Can you work these out from the model? Positions are in its coordinate system, mm. Face numbers are marked on the shaded views. A direction names the side the tool comes from. Coordinates: 2 decimals unless noted, no trailing zeros. Write each loop counter-clockwise with the first axis right and the second up, starting at its lowest first coordinate (ties: lowest second). Pieces come first, ordered by that corner, then holes.
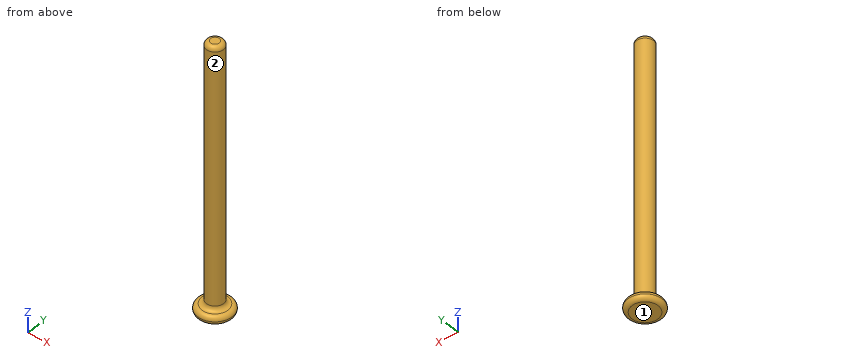
Autodesk Inventor part; units mm, degrees
ref_plane "YZ Plane" through (0, 0, 0) normal (1, 0, 0) x (0, 1, 0)
ref_plane "XZ Plane" through (0, 0, 0) normal (0, 1, 0) x (-1, 0, 0)
ref_plane "XY Plane" through (0, 0, 0) normal (0, 0, 1) x (1, 0, 0)
sketch "Sketch1" plane through (0, 0, 0) normal (0, 0, 1) x (1, 0, 0)
  circle A0 centre (0, 0) radius 2
  dimension "d0" = 4
extrude "Extrusion1" add sketch "Sketch1" along normal blind 1
sketch "Sketch2" plane through (0, 0, 1) normal (0, 0, 1) x (1, 0, 0)
  circle A0 centre (0, 0) radius 1
  dimension "d3" = 2
extrude "Extrusion2" add sketch "Sketch2" along normal blind 30
fillet "Fillet1" radius 0.5 1 edges at (-1, 0, 31)
fillet "Fillet2" radius 0.5 3 edges at (-1, 0, 1) (-2, 0, 1) (-2, 0, 0)
properties part number "ufakpin"
1. If I drill on L1, parallel to Y at x = -0.1, z = 23.5; L2, parallel to Z at x = 1.2, y = -0.75; L3, parallel to Z at x = 1.15, y = -0.2, over which ranges is the centre line in solid material (lowest first)?
2. Which directions (+Z, -Z, +X, -X, +Y, -Y) give clear straight access to the entire face, cutting with the end or side of a thin tool? Please do the marked faces 1 and 2.
3. If we section it at A-A, the plane z = 21.5: List the corners of the cut face in (x, y) for me, plus the area to 3 significant figures.
4. I'm going to push a flat-ended pin straight in: P1, Ø2, axis at x = -1, y = -1.5, coming from the +Z side. Where does the tip first touch, or does it pass through?
Answers:
1. L1: y = -0.99 to 0.99
1. L2: z = 0 to 1.01
1. L3: z = 0 to 1.13
2. face 1: -Z, +X, -X, +Y, -Y
2. face 2: +Z
3. outline: circle Ø2 at (0, 0)
3. area: 3.14 mm2
4. P1: stops at z = 30.9
